Here's the drawing with two shaded views (mm, measured from the low corner). I have some questions. Coordinates: 2 decimals unless noted, no trailing zeros. Write each loop counter-clockwise with the first axis right and the second up, starting at its lowest first coordinate (ties: lowest second). Pieces come first, ordered by that corner, then holes.
Item 1: I want a section at C-C on z = 33.5. Please give me the cut outline in (x, y).
Item 2: I want a section at A-A on z = 25.5. Please give me the cut outline in (x, y), then the cut area to 3 significant figures.
Item 3: I want a section at B-B on z = 4.5. Please give me the cut outline in (x, y).
Item 4: Thinking about a two-plate mould opening in Y: for the marked faces 1, 2 and 3, which applies, +Y half, -Y half, draft (parallel to the pull), parting line (faces both ways), or undercut?
Item 5: For P1, Ø8, axis at x = 58.5, z = 22.5, coming from the +Y side; P2, Ø1, axis at x = 50, y = 43, coming from the +Z side; P3, Ø3, axis at x = 50, z = 4.5, coming from the -Y side, each with a flat end and sliding along its axis, tell me the tip position at first contact or that it passes through.
Item 6: If I drill on probe 1 along X at (y, z) = (35, 13.1); probe 2 along Y at (x, z) = (36.5, 9); probe 3 along X at (y, z) = (35, 12.95), over which ranges is the centre line in solid material (lowest first)?
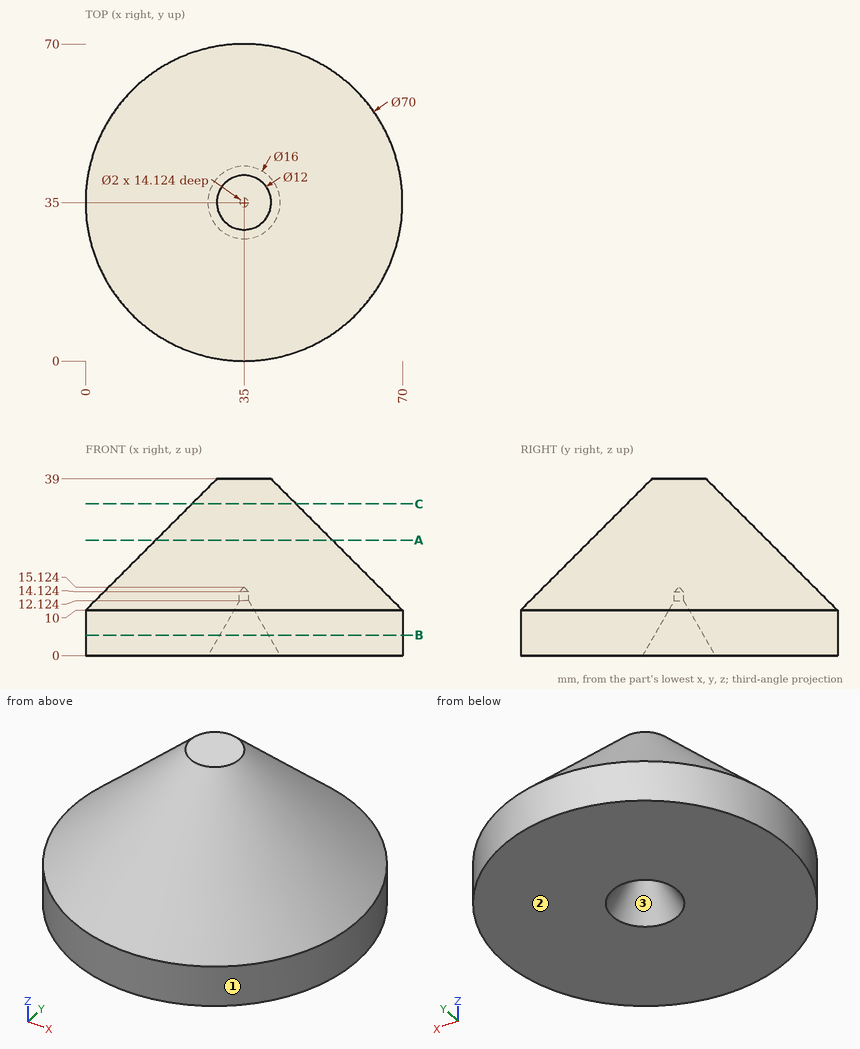
Response values:
1. outline: circle Ø23 at (35, 35)
2. outline: circle Ø39 at (35, 35)
2. area: 1,190 mm2
3. outline: circle Ø70 at (35, 35); hole circle Ø10.8 at (35, 35)
4. face 1: parting line
4. face 2: draft
4. face 3: undercut
5. P1: stops at y = 49.68
5. P2: stops at z = 28.5
5. P3: stops at y = 2.71
6. probe 1: x = 3.1 to 34, 36 to 66.9
6. probe 2: y = 0.03 to 32.63, 37.37 to 69.97
6. probe 3: x = 2.95 to 34, 36 to 67.05
